Source: CAD feature listing. Evaluate the final solid. Frame: model axes, mm. A direction names the side the tool comes from. Give positions to 0.01 mm unless a question says otherwise; leave off trailing zeros. Order: outer loops, then holes, each group sorted by start corner. A loop starts at its lowest first (then second) coordinate and runs counter-clockwise, first axis right, second up. Notation, with made-up numbers: (-30, 56.5) -> (17, 56.5) arc R17 cw to (17, 76.5) -> close; hole circle Ø3 at (9, 50.25). An arc over 180 degrees is marked (long way). Answer in a Markdown table with one row per item.
```python
from build123d import *

# Parameters (mm, degrees)
SKETCH1_W             = 70
SKETCH1_H             = 30
SKETCH1_R             = 4.5
SKETCH1_R_2           = 1.495
SKETCH1_R_3           = 0.995
SKETCH1_R_4           = 2
BOSS_EXTRUDE1_DEPTH   = 4.5
F_2_CLEARANCE_HOLE1_D = 2.2606
SKETCH6_R             = 7
CUT_EXTRUDE1_DEPTH    = 3.5
SKETCH7_R             = 3.5
SKETCH7_R_2           = 1.495
BOSS_EXTRUDE2_DEPTH   = 2
SKETCH8_R             = 2
SKETCH8_R_2           = 0.995
BOSS_EXTRUDE3_DEPTH   = 2


with BuildPart() as part:
    # Sketch1 → Boss-Extrude1 (new body)
    with BuildSketch(Plane.XY):
        with Locations((20, 0)):
            Rectangle(SKETCH1_W, SKETCH1_H)
        Circle(SKETCH1_R, mode=Mode.SUBTRACT)
        with Locations((18.05, 0)):
            Circle(SKETCH1_R_2, mode=Mode.SUBTRACT)
        with Locations((32.6, 0)):
            Circle(SKETCH1_R_3, mode=Mode.SUBTRACT)
        with Locations((42.449999958, 0)):
            Circle(SKETCH1_R_4, mode=Mode.SUBTRACT)
    extrude(amount=BOSS_EXTRUDE1_DEPTH)

    # #2 Clearance Hole1 (through all)
    with Locations(Plane.XY.offset(4.5)):
        with Locations((-12.5, 12.5), (-12.5, -12.5), (27.5, 12.5), (27.5, -12.5), (52.5, 12.5), (52.5, -12.5)):
            Hole(F_2_CLEARANCE_HOLE1_D / 2)

    # Sketch6 → Cut-Extrude1 (cut)
    with BuildSketch(Plane.XY.offset(4.5)):
        Circle(SKETCH6_R)
    extrude(amount=-CUT_EXTRUDE1_DEPTH, mode=Mode.SUBTRACT)

    # Sketch7 → Boss-Extrude2 (add)
    with BuildSketch(Plane.XY.offset(4.5)):
        with Locations((18.05, 0)):
            Circle(SKETCH7_R)
        with Locations((18.05, 0)):
            Circle(SKETCH7_R_2, mode=Mode.SUBTRACT)
    extrude(amount=BOSS_EXTRUDE2_DEPTH)

    # Sketch8 → Boss-Extrude3 (add)
    with BuildSketch(Plane.XY.offset(4.5)):
        with Locations((32.6, 0)):
            Circle(SKETCH8_R)
        with Locations((32.6, 0)):
            Circle(SKETCH8_R_2, mode=Mode.SUBTRACT)
    extrude(amount=BOSS_EXTRUDE3_DEPTH)


solid = part.part
```
(1) Access query for faces 4 (the cylindrical face through (-0.59, 4.46, 0.49)), 5 (the cylindrical face through (6.466, -2.681, 2.774)). Directions: +Z, -Z, +X, -X, +Y, -Y. A direction counts if a zero-diameter tool reaches every point of the face in a straight line with its end or side. Return the directions, or none.
A:
| item | result |
|---|---|
| face 4 | +Z, -Z |
| face 5 | +Z |
(2) Section query B-B (x = 18.05). Return the cut outline in (y, z) (3 decimals).
A:
| item | result |
|---|---|
| outline | (-15, 0) -> (-1.495, 0) -> (-1.495, 6.5) -> (-3.5, 6.5) -> (-3.5, 4.5) -> (-15, 4.5) -> close; (1.495, 0) -> (15, 0) -> (15, 4.5) -> (3.5, 4.5) -> (3.5, 6.5) -> (1.495, 6.5) -> close |
(3) Ray query, probe 1 along Y at (x, z) = (52.5, 2.3); probe 2 along X at (y, z) = (0.25, 2); probe 3 along Y at (x, z) = (42.45, 2.75). Return the intervals inside material, ascending.
A:
| item | result |
|---|---|
| probe 1 | y = -15 to -13.63, -11.37 to 11.37, 13.63 to 15 |
| probe 2 | x = -15 to -7, 7 to 16.58, 19.52 to 31.64, 33.56 to 40.47, 44.43 to 55 |
| probe 3 | y = -15 to -2, 2 to 15 |
(4) First-contact query: pin 1 Ø1 at (x, y) = (-1.5, -11) entering from +Z; pin 2 Ø10.5 at (x, y) = (0, 0) entering from +Z; pin 3 Ø2.5 at (x, y) = (27.5, -12.5) entering from -Z. Flat tips, straight axial feed; report the tip coordinate or a pass-through.
A:
| item | result |
|---|---|
| pin 1 | stops at z = 4.5 |
| pin 2 | stops at z = 1 |
| pin 3 | stops at z = 0 |
(5) Section query A-A (y = 0). Give the number of separate pieces and of enclosed holes in the cut face, plus the area to 3 significant figures.
A:
| item | result |
|---|---|
| separate pieces | 5 |
| enclosed holes | 0 |
| area | 229 mm^2 |
(6) Section query C-C (y = 12.5). Return the cut outline in (x, z), plus the area to 3 significant figures.
A:
| item | result |
|---|---|
| outline | (-15, 0) -> (-13.63, 0) -> (-13.63, 4.5) -> (-15, 4.5) -> close; (-11.37, 0) -> (26.37, 0) -> (26.37, 4.5) -> (-11.37, 4.5) -> close; (28.63, 0) -> (51.37, 0) -> (51.37, 4.5) -> (28.63, 4.5) -> close; (53.63, 0) -> (55, 0) -> (55, 4.5) -> (53.63, 4.5) -> close |
| area | 284 mm^2 |
(7) Pull-direction query (X, two-part tool) for faces 1 (the flat face through (55, 0, 2)), 2 (the flat face through (-15, 0, 2)), 3 (the cylindrical face through (51.42, 12.84, 2.22)); classes: +X half, -X half, draft (parallel to the pull), parting line (faces both ways), or undercut.
A:
| item | result |
|---|---|
| face 1 | +X half |
| face 2 | -X half |
| face 3 | undercut |
